Read the model definition and answer for the solid it produces. Units are mm, in the model's axes. A direction names the side the tool comes from. Give positions to 0.01 mm unless a question says otherwise; leave off trailing zeros. Loops run counter-clockwise (first coordinate to the right, second up) from the corner with the lowest first, then second, coordinate; pieces in that order, holes last. Notation, with made-up numbers: (11, 83.5) - (47, 83.5) arc R5 ccw to (47, 89.5) - close; hole circle Ø3 at (34.25, 86.5). An arc over 180 degrees is marked (long way). Write item = value, one per line.
```python
from build123d import *

# Parameters (mm, degrees)
SKETCH1_W           = 93.98
SKETCH1_H           = 19.05
BOSS_EXTRUDE1_DEPTH = 2.6289
SKETCH2_W           = 93.98
SKETCH2_H           = 25.4
BOSS_EXTRUDE2_DEPTH = 5.2578
FILLET6_R           = 4.572
FILLET7_R           = 4.572
FILLET8_R           = 1.524
FILLET9_R           = 2.54
FILLET10_R          = 2.54
CAVITY1_START       = 9.525
CAVITY1_OUTLINE_R   = 1.7526
CAVITY1_DEPTH       = 5.2578


# Read off the part's stored shape, not the designer's step: Cavity1
with BuildPart() as part:
    # Sketch1 → Boss-Extrude1 (new, symmetric)
    with BuildSketch(Plane.XY):
        Rectangle(SKETCH1_W, SKETCH1_H)
    extrude(amount=BOSS_EXTRUDE1_DEPTH, both=True)

    # Sketch2 → Boss-Extrude2 (add)
    with BuildSketch(Plane(origin=(0, 9.525, 0), x_dir=(1, 0, 0), z_dir=(0, 1, 0))):
        with Locations((0, 10.0711)):
            Rectangle(SKETCH2_W, SKETCH2_H)
    extrude(amount=BOSS_EXTRUDE2_DEPTH)

    # Fillet6
    fillet6_edges = [part.edges().sort_by_distance(p)[0] for p in [
        (-46.99, -9.525, 0),
    ]]
    fillet(fillet6_edges, radius=FILLET6_R)

    # Fillet7
    fillet7_edges = [part.edges().sort_by_distance(p)[0] for p in [
        (46.99, -9.525, 0),
    ]]
    fillet(fillet7_edges, radius=FILLET7_R)

    # Fillet8
    fillet8_edges = [part.edges().sort_by_distance(p)[0] for p in [
        (0, 14.7828, 2.6289),
    ]]
    fillet(fillet8_edges, radius=FILLET8_R)

    # Fillet9
    fillet9_edges = [part.edges().sort_by_distance(p)[0] for p in [
        (-46.99, 12.1539, -22.7711),
    ]]
    fillet(fillet9_edges, radius=FILLET9_R)

    # Fillet10
    fillet10_edges = [part.edges().sort_by_distance(p)[0] for p in [
        (46.99, 12.1539, -22.7711),
    ]]
    fillet(fillet10_edges, radius=FILLET10_R)

    # Cavity1 outline → Cavity1 (cut)
    with BuildSketch(Plane(origin=(0, 0, 0), x_dir=(1, 0, 0), z_dir=(0, 1, 0)).offset(CAVITY1_START)):
        with Locations((25.019, 12.7)):
            Circle(CAVITY1_OUTLINE_R)
        with Locations((-11.5062, 12.7)):
            Circle(CAVITY1_OUTLINE_R)
    extrude(amount=CAVITY1_DEPTH, mode=Mode.SUBTRACT)


solid = part.part
```
1) Each of these flat-tipped pins is pushed along its axis until it touches: P1, Ø5, axis at y = -3, z = -4.5, coming from the +X side; P2, Ø2, axis at x = 35.5, y = 2.5, coming from the -Z side. Where does it stop, or does it pass through?
Output:
P1 = 46.99
P2 = -2.63
2) A cutting plane is placed at D-D on y = -6.75. Determine the outline of the cut face in (x, z).
Output:
outline = (-46.62, -2.63) - (46.62, -2.63) - (46.62, 2.63) - (-46.62, 2.63) - close
3) A cutting plane is placed at A-A on z = -12.7. Determine the outline of the cut face in (x, y) (3 decimals), then the cut area to 3 significant figures.
Output:
outline = (-46.99, 9.525) - (-13.259, 9.525) - (-13.259, 14.783) - (-46.99, 14.783) - close; (-9.754, 9.525) - (23.266, 9.525) - (23.266, 14.783) - (-9.754, 14.783) - close; (26.772, 9.525) - (46.99, 9.525) - (46.99, 14.783) - (26.772, 14.783) - close
area = 457 mm²
4) Find the intervals of material crossed by probe 1 along X at (y, z) = (12.5, -12.7); probe 2 along Z at (x, y) = (29, 6); probe 3 along Y at (x, z) = (-37, -18) (3 decimals), in increasing order.
Output:
probe_1 = -46.99 to -13.26, -9.75 to 23.27, 26.77 to 46.99
probe_2 = -2.63 to 2.63
probe_3 = 9.525 to 14.783
5) A cutting plane is placed at B-B on x = 2. Determine the outline of the cut face in (y, z) (3 decimals), then the cut area to 3 significant figures.
Output:
outline = (-9.525, -2.629) - (9.525, -2.629) - (9.525, -22.771) - (14.783, -22.771) - (14.783, 1.105) arc R1.524 ccw to (13.259, 2.629) - (-9.525, 2.629) - close
area = 233 mm²
6) A tool of negligible diameter and unlimited length cuts with its end or side. For faces 1 (the face through (-1, 9.525, -13)), 2 (the face through (-1, 2, 2.629)), from which of +Z, -Z, +X, -X, +Y, -Y can it reach the whole face along a straight path? Write none if from no direction.
Output:
face_1 = -Z, +X, -X, -Y
face_2 = +Z, +X, -X, +Y, -Y
7) A cutting plane is placed at C-C on y = 8.5. Determine the outline of the cut face in (x, z), then the cut area to 3 significant figures.
Output:
outline = (-46.99, -2.63) - (46.99, -2.63) - (46.99, 2.63) - (-46.99, 2.63) - close
area = 494 mm²
